Drawing for the job (mm, zero at the part's lowest x, y, z). A direction names the side the tool comes from. Give positions to 0.01 mm unless a question says otherwise; leave off trailing zeros. Write each loop counter-clockwise with the first axis right and the second up, starting at its lowest first coordinate (ties: lowest second). Pieces come first, ordered by that corner, then holes. Notation, with made-up numbers: (-27, 52) - (-10, 52) arc R7 cw to (-10, 62) - close; hole circle Ø1 at (-8.75, 16.5). An arc over 180 degrees is marked (long way). Use CSV: the item, a comma, the result in double quotes.
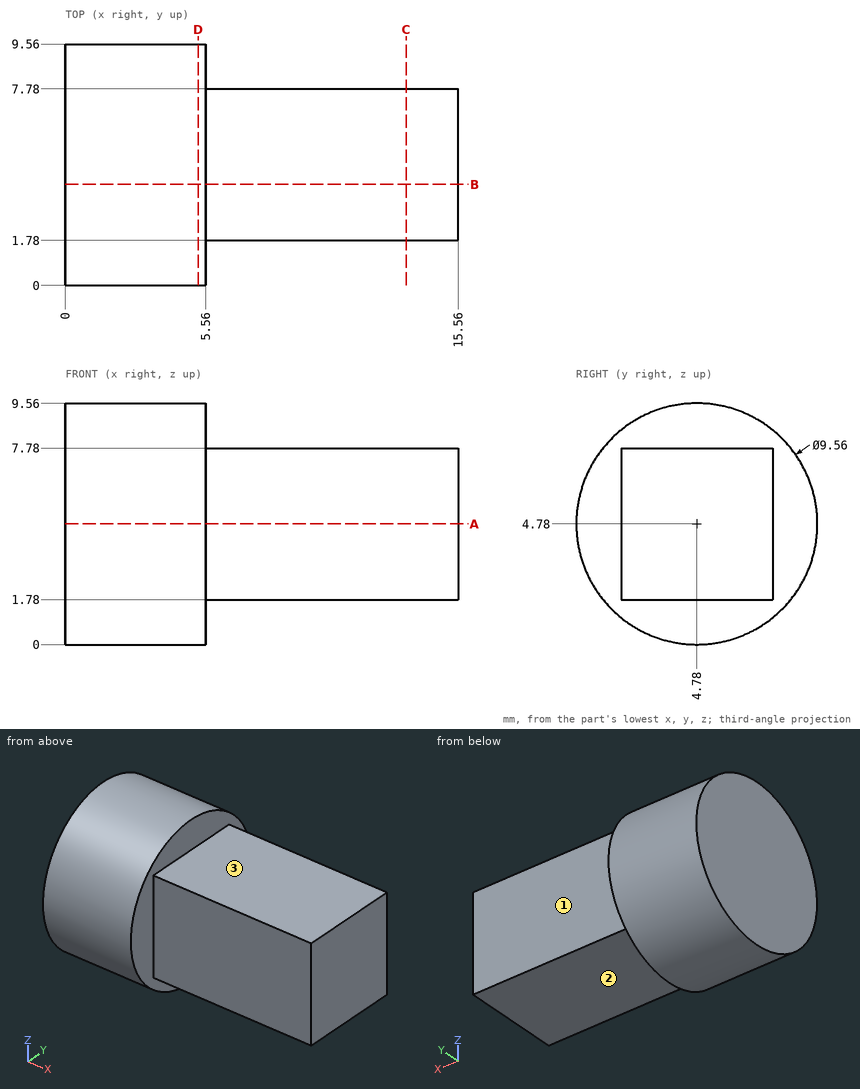
(1) Saw through at A-A, the plane z = 4.78. List the corners of the cut face in (x, y), then the cut area to 3 significant figures.
Checked values:
outline,"(0, 0) - (5.56, 0) - (5.56, 1.78) - (15.56, 1.78) - (15.56, 7.78) - (5.56, 7.78) - (5.56, 9.56) - (0, 9.56) - close"
area,"113 mm^2"
(2) Saw through at B-B, the plane y = 4. List the corners of the cut face in (x, z), then the cut area to 3 significant figures.
Checked values:
outline,"(0, 0.06) - (5.56, 0.06) - (5.56, 1.78) - (15.56, 1.78) - (15.56, 7.78) - (5.56, 7.78) - (5.56, 9.5) - (0, 9.5) - close"
area,"112 mm^2"
(3) Saw through at C-C, the plane x = 13.5. List the corners of the cut face in (y, z), then the cut area to 3 significant figures.
Checked values:
outline,"(1.78, 1.78) - (7.78, 1.78) - (7.78, 7.78) - (1.78, 7.78) - close"
area,"36.0 mm^2"
(4) Flat gauge pins, fed straight in: P1, Ø5, axis at x = 10.5, z = 4, coming from the -Y side; P2, Ø2, axis at x = 12.5, z = 3.5, coming from the +Y side; P3, Ø3, axis at x = 10.5, y = 4.5, coming from the +Z side. Where does each tip first touch, or does it go through?
Checked values:
P1,"stops at y = 1.78"
P2,"stops at y = 7.78"
P3,"stops at z = 7.78"
(5) Saw through at D-D, the plane x = 5.25. List the corners of the cut face in (y, z).
Checked values:
outline,"circle Ø9.56 at (4.78, 4.78)"
(6) 3-axis set-ups, long thin cutter, end or side, ignore diameter. For the marked faces 1, 2 and 3: which of +Z, -Z, +X, -X, +Y, -Y reach the whole face in a straight line?
Checked values:
face 1,"+Z, -Z, +X, +Y"
face 2,"-Z, +X, +Y, -Y"
face 3,"+Z, +X, +Y, -Y"
(7) Wall check: probe 1 along X at (y, z) = (2.5, 1); probe 2 along Z at (x, y) = (12.5, 2). Give the ranges that are in metal, low to high. Write a range as [from, to].
Checked values:
probe 1,"x = [0, 5.56]"
probe 2,"z = [1.78, 7.78]"
